from build123d import *

# Parameters (mm, degrees)
SKETCH_1_W                  = 5
SKETCH_1_H                  = 60
EXTRUDE_2_DEPTH             = 60
SKETCH_2_R                  = 5
SKETCH_3_R                  = 3.5
CUT_EXTRUDE_1_DEPTH         = 137.839321834
HOLE_WIZARD_M81_D           = 9
HOLE_WIZARD_M81_CSINK_D     = 17.3
HOLE_WIZARD_M81_CSINK_ANGLE = 90


with BuildPart() as part:
    # Эскиз1 → Вытянуть-Тонкостенный2 (new, symmetric)
    with BuildSketch(Plane.XY):
        with Locations((2.5, 30)):
            Rectangle(SKETCH_1_W, SKETCH_1_H)
    extrude(amount=EXTRUDE_2_DEPTH, both=True)

    # По траектории1: sweep along a curve in space
    with BuildLine() as sweep_1_path:
        Line((0, 60, 60), (0, 60, -60))
    # Эскиз2 → По траектории1 (sweep)
    with BuildSketch(Plane.XY.offset(60)):
        with Locations((5, 60)):
            Circle(SKETCH_2_R)
    sweep(path=sweep_1_path.line)

    # Эскиз3 → Вырез-Вытянуть1 (cut, through all)
    with BuildSketch(Plane.XY.offset(60)):
        with Locations((5, 60)):
            Circle(SKETCH_3_R)
    extrude(amount=-CUT_EXTRUDE_1_DEPTH, mode=Mode.SUBTRACT)

    # Зенковка для  винта с плоской головкой M81 (through all)
    with Locations(Plane(origin=(0, 0, 0), x_dir=(0, 0, -1), z_dir=(-1, 0, 0))):
        with Locations((-45, -30), (-20, -15)):
            hole_wizard_m81 = CounterSinkHole(HOLE_WIZARD_M81_D / 2, HOLE_WIZARD_M81_CSINK_D / 2, counter_sink_angle=HOLE_WIZARD_M81_CSINK_ANGLE)

    # Зеркальное отражение4: Зенковка для  винта с плоской головкой M81 across plane
    add(hole_wizard_m81.mirror(Plane.XY), mode=Mode.SUBTRACT)


solid = part.part
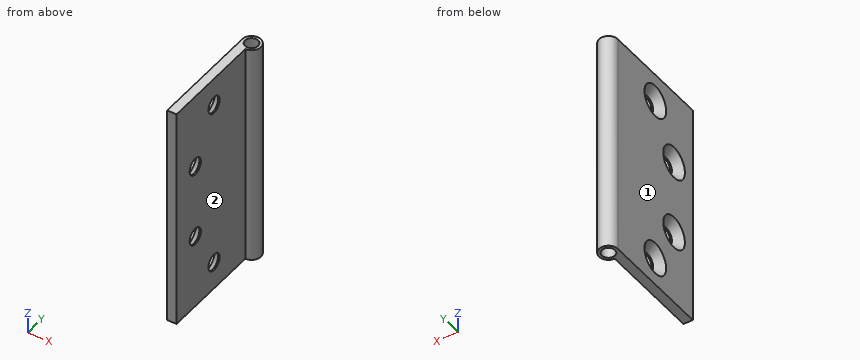
The listing builds one solid part. Answer for the finished solid, in the listing's coordinates (mm). Face numbers are marked on the shaded views. A direction names the side the tool comes from. Give positions to 0.01 mm unless a question says otherwise; leave off trailing zeros. Write each loop counter-clockwise with the first axis right and the second up, starting at its lowest first coordinate (ties: lowest second). Pieces come first, ordered by that corner, then holes.
Item 1: Section B-B, the plane z = -20 is taken. Write down the section's boundary in (x, y).
Item 2: Which of the six approach directions +Z, -Z, +X, -X, +Y, -Y give full straight-line access (tool end or side, diameter ignored) to the marked faces 1 and 2?
Item 3: Flat-ended cylindrical pins translate along their axes: P1, Ø1, axis at y = 55.5, z = 47, coming from the +X side; P2, Ø11.5, axis at y = 15, z = 20, coming from the -X side; P3, Ø8, axis at y = 31.5, z = 45.5, coming from the -X side. Find the tip coordinate at first contact, or state that the pin passes through.
Item 4: Section C-C, the plane z = 1 is taken. Write down the section's boundary in (x, y).
Item 5: Section A-A, the plane y = 30 is taken. Write down the section's boundary in (x, z).
Item 6: Find the intervals of material crossed by line 1 along Y through (x, z) = (4.7, 45); line 2 along X through (y, z) = (8, -47); line 3 along Y through (x, z) = (7, -9), in increasing order.
Item 7: Section D-D, the plane y = 40 is taken. Write down the section's boundary in (x, z).
Completed:
1. outline: (0, 0) - (5, 0) - (5, 10.5) - (4.15, 10.5) - (0, 6.35) - close; (0, 23.65) - (4.15, 19.5) - (5, 19.5) - (5, 55) arc R5 ccw (long way) to (0, 60) - close; hole circle Ø7 at (5, 60)
2. face 1: +Z, -Z, -X, +Y, -Y
2. face 2: +Z, -Z, +X, -Y
3. P1: stops at x = 8
3. P2: stops at x = 2.9
3. P3: stops at x = 3.07
4. outline: (0, 0) - (5, 0) - (5, 55) arc R5 ccw (long way) to (0, 60) - close; hole circle Ø7 at (5, 60)
5. outline: (0, -60) - (5, -60) - (5, -49.5) - (4.15, -49.5) - (0, -53.65) - close; (0, -36.35) - (4.15, -40.5) - (5, -40.5) - (5, 40.5) - (4.15, 40.5) - (0, 36.35) - close; (0, 53.65) - (4.15, 49.5) - (5, 49.5) - (5, 60) - (0, 60) - close
6. line 1: y = 0 to 25.5, 34.5 to 56.51, 63.49 to 64.99
6. line 2: x = 0 to 5
6. line 3: y = 55.42 to 57.13, 62.87 to 64.58
7. outline: (0, -60) - (5, -60) - (5, 60) - (0, 60) - close
